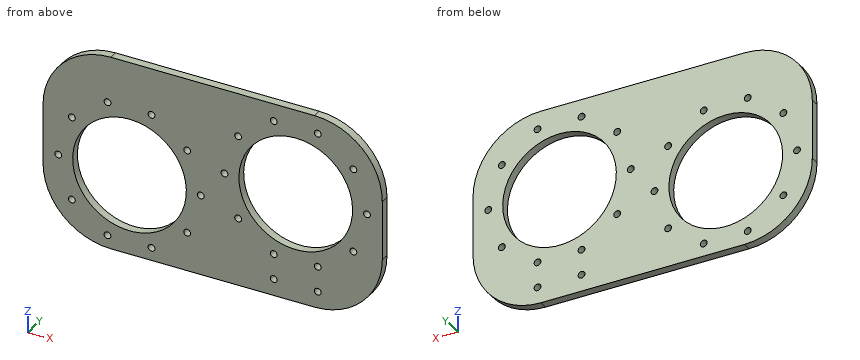
```python
from build123d import *

# Parameters (mm, degrees)
SKETCH_1_R               = 33.5
EXTRUDE_1_DEPTH          = 5
CUT_EXTRUDE_1_REACH      = 117.461
SKETCH_2_R               = 2
PATTERN_CIRCULAR_1_COUNT = 10
CUT_EXTRUDE_2_REACH      = 117.461
SKETCH_3_R               = 2
PATTERN_CIRCULAR_2_COUNT = 10
CUT_EXTRUDE_3_REACH      = 117.461
SKETCH_4_R               = 2


with BuildPart() as part:
    # 草圖1 → 填料-伸長1 (new body)
    with BuildSketch(Plane(origin=(0, 0, 0), x_dir=(1, 0, 0), z_dir=(0, 1, 0))):
        with BuildLine():
            Line((-60, 57.5), (60, 57.5))
            ThreePointArc((60, 57.5), (88.284271247, 45.784271247), (100, 17.5))
            Line((100, 17.5), (100, -17.5))
            ThreePointArc((100, -17.5), (88.284271247, -45.784271247), (60, -57.5))
            Line((60, -57.5), (-60, -57.5))
            ThreePointArc((-60, -57.5), (-88.284271247, -45.784271247), (-100, -17.5))
            Line((-100, -17.5), (-100, 17.5))
            ThreePointArc((-100, 17.5), (-88.284271247, 45.784271247), (-60, 57.5))
        make_face()
        with Locations(Location((-49, 10, 0), (0, 0, 270))):
            Circle(SKETCH_1_R, mode=Mode.SUBTRACT)
        with Locations(Location((49, -7.280044109, 0), (0, 0, 270))):
            Circle(SKETCH_1_R, mode=Mode.SUBTRACT)
    extrude(amount=EXTRUDE_1_DEPTH)

    # 草圖2 → 除料-伸長1 (cut, up to next)
    with BuildSketch(Plane(origin=(0, 5, 0), x_dir=(1, 0, 0), z_dir=(0, 1, 0)), mode=Mode.PRIVATE) as cut_extrude_1_sk1:
        with Locations(Location((91, -7.280044109, 0), (0, 0, 270))):
            Circle(SKETCH_2_R)
    cut_extrude_1_tool1 = extrude(cut_extrude_1_sk1.sketch, amount=-CUT_EXTRUDE_1_REACH, mode=Mode.PRIVATE) & part.part
    cut_extrude_1 = cut_extrude_1_tool1.solids().sort_by_distance((91, 5, 7.280044))[0]
    add(cut_extrude_1, mode=Mode.SUBTRACT)

    # 環狀複製排列1: 除料-伸長1 ×10 about axis
    pattern_circular_1_axis = Axis((49, 0, 7.280044109), (0, 1, 0))
    for i in range(1, PATTERN_CIRCULAR_1_COUNT):
        add(cut_extrude_1.rotate(pattern_circular_1_axis, i * 360 / PATTERN_CIRCULAR_1_COUNT), mode=Mode.SUBTRACT)

    # 草圖3 → 除料-伸長2 (cut, up to next)
    with BuildSketch(Plane(origin=(0, 5, 0), x_dir=(1, 0, 0), z_dir=(0, 1, 0)), mode=Mode.PRIVATE) as cut_extrude_2_sk1:
        with Locations(Location((-7, 10, 0), (0, 0, 270))):
            Circle(SKETCH_3_R)
    cut_extrude_2_tool1 = extrude(cut_extrude_2_sk1.sketch, amount=-CUT_EXTRUDE_2_REACH, mode=Mode.PRIVATE) & part.part
    cut_extrude_2 = cut_extrude_2_tool1.solids().sort_by_distance((-7, 5, -10))[0]
    add(cut_extrude_2, mode=Mode.SUBTRACT)

    # 環狀複製排列2: 除料-伸長2 ×10 about axis
    pattern_circular_2_axis = Axis((-49, 0, -10), (0, 1, 0))
    for i in range(1, PATTERN_CIRCULAR_2_COUNT):
        add(cut_extrude_2.rotate(pattern_circular_2_axis, i * 360 / PATTERN_CIRCULAR_2_COUNT), mode=Mode.SUBTRACT)

    # 草圖4 → 除料-伸長3 (cut, up to next)
    with BuildSketch(Plane(origin=(0, 5, 0), x_dir=(1, 0, 0), z_dir=(0, 1, 0)), mode=Mode.PRIVATE) as cut_extrude_3_sk1:
        with Locations(Location((36.021286236, 47.664329575, 0), (0, 0, 270))):
            Circle(SKETCH_4_R)
    cut_extrude_3_tool1 = extrude(cut_extrude_3_sk1.sketch, amount=-CUT_EXTRUDE_3_REACH, mode=Mode.PRIVATE) & part.part
    # 草圖4 → 除料-伸長3 (cut, up to next)
    with BuildSketch(Plane(origin=(0, 5, 0), x_dir=(1, 0, 0), z_dir=(0, 1, 0)), mode=Mode.PRIVATE) as cut_extrude_3_sk2:
        with Locations(Location((61.978713764, 47.664329575, 0), (0, 0, 270))):
            Circle(SKETCH_4_R)
    cut_extrude_3_tool2 = extrude(cut_extrude_3_sk2.sketch, amount=-CUT_EXTRUDE_3_REACH, mode=Mode.PRIVATE) & part.part
    add(cut_extrude_3_tool1.solids().sort_by_distance((36.021286, 5, -47.66433))[0], mode=Mode.SUBTRACT)
    add(cut_extrude_3_tool2.solids().sort_by_distance((61.978714, 5, -47.66433))[0], mode=Mode.SUBTRACT)


solid = part.part
```
Source: CAD feature listing. Evaluate the final solid. Frame: model axes, mm. Round coordinates to 2 decimals unless told otherwise and drop trailing zeros. Loops run counter-clockwise (first coordinate to the right, second up) from the corner with the lowest first, then second, coordinate; pieces in that order, holes last. Notation, with made-up numbers: M -32.5,86 L 13.5,86 A26 ccw 13.5,120 Z; hole C 88.25,-35.75 d3. An arc over 180 degrees is marked long. Use a Markdown table: item, result. Add a question column.
1. Contact query for a flat-ended pin moving along its axis: P1, Ø5, axis at x = -48.5, z = -39.5, coming from the +Y side. Output: stop coordinate, or through.
2. Section query C-C on y = 1.65. Give the number of separate pieces and of enclosed holes in the cut face, then the cut area to 3 significant figures.
3. Section query B-B on z = -10. Return the cut outline in (x, y).
4. Section query D-D on x = -49. Return the cut outline in (y, z), then the cut area to 3 significant figures.
5. Line query: line 1 (X direction, y = 4.4, z = 7); line 2 (X direction, y = 1.05, z = 31); line 3 (X direction, y = 1.6, z = -16.5). Output: solid intervals per line, ascending.
6. Section query A-A on x = -7. Return the cut outline in (y, z), then the cut area to 3 significant figures.
Reported:
| question | item | result |
|---|---|---|
| 1 | P1 | passes through |
| 2 | separate pieces | 1 |
| 2 | enclosed holes | 24 |
| 2 | area | 14,300 mm² |
| 3 | outline | M -100,0 L -93,0 L -93,5 L -100,5 Z; M -89,0 L -82.5,0 L -82.5,5 L -89,5 Z; M -15.5,0 L -9,0 L -9,5 L -15.5,5 Z; M -5,0 L 20.3,0 L 20.3,5 L -5,5 Z; M 77.7,0 L 100,0 L 100,5 L 77.7,5 Z |
| 4 | outline | M 0,-57.5 L 5,-57.5 L 5,-43.5 L 0,-43.5 Z; M 0,23.5 L 5,23.5 L 5,57.5 L 0,57.5 Z |
| 4 | area | 240 mm² |
| 5 | line 1 | x = -100 to -77.87, -20.13 to 5.02, 8.98 to 15.5, 82.5 to 89.02, 92.98 to 100 |
| 5 | line 2 | x = -97.65 to -63.68, -60.28 to -37.72, -34.32 to 13.27, 16.77 to 25.34, 72.66 to 81.23, 84.73 to 97.65 |
| 5 | line 3 | x = -100 to -81.86, -16.14 to 13.24, 16.8 to 25.4, 72.6 to 81.2, 84.76 to 100 |
| 6 | outline | M 0,-57.5 L 5,-57.5 L 5,-12 L 0,-12 Z; M 0,-8 L 5,-8 L 5,57.5 L 0,57.5 Z |
| 6 | area | 555 mm² |
